Source: CAD feature listing. Evaluate the final solid. Frame: model axes, mm. A direction names the side the tool comes from. Give positions to 0.01 mm unless a question says otherwise; leave off trailing zeros. Order: outer loops, then holes, each group sorted by start corner. A loop starts at its lowest first (then second) coordinate and runs counter-clockwise, first axis right, second up. Notation, with made-up numbers: (-9, 21.5) - (14, 21.5) arc R12 cw to (14, 25.5) - close; hole circle Ø5 at (69.5, -11). An arc over 180 degrees is marked (long way). Answer as CSV lines item,"result".
```python
from build123d import *

# Parameters (mm, degrees)
SKETCH_W             = 47.4
SKETCH_H             = 2
PAD_DEPTH            = 10
SKETCH002_W          = 12
SKETCH002_H          = 10
PAD001_DEPTH         = 2.75
SKETCH003_R          = 1.65
POCKET_DEPTH         = 2.001
POCKET_DEPTH_BACK    = 2.751
POCKET001_DEPTH      = 2.001
POCKET001_DEPTH_BACK = 2.751


with BuildPart() as part:
    # Sketch → Pad (new body)
    with BuildSketch(Plane.XY):
        with Locations((0, 1)):
            Rectangle(SKETCH_W, SKETCH_H)
    extrude(amount=-PAD_DEPTH)

    # Sketch002 → Pad001 (join)
    with BuildSketch(Plane.XZ):
        with Locations((-6.6, -5)):
            Rectangle(SKETCH002_W, SKETCH002_H)
        with Locations((6.6, -5)):
            Rectangle(SKETCH002_W, SKETCH002_H)
    extrude(amount=PAD001_DEPTH)

    # Sketch003 → Pocket (cut, two sides)
    with BuildSketch(Plane.XZ) as pocket_sk:
        with Locations((-14.75, -5)):
            Circle(SKETCH003_R)
        with Locations((14.75, -5)):
            Circle(SKETCH003_R)
    extrude(amount=-POCKET_DEPTH, mode=Mode.SUBTRACT)
    extrude(pocket_sk.sketch, amount=POCKET_DEPTH_BACK, mode=Mode.SUBTRACT)

    # Sketch004 → Pocket001 (cut, two sides)
    with BuildSketch(Plane.XZ) as pocket001_sk:
        Polygon((-18.2, 0), (-23.7, -5.5), (-23.7, 0), align=None)
        Polygon((18.2, 0), (23.7, 0), (23.7, -5.5), align=None)
    extrude(amount=-POCKET001_DEPTH, mode=Mode.SUBTRACT)
    extrude(pocket001_sk.sketch, amount=POCKET001_DEPTH_BACK, mode=Mode.SUBTRACT)


solid = part.part
```
(1) Mould query, pull axis X, two halves, no side actions, for faces 4 (the flat face through (-12.6, -1, -5)), 5 (the flat face through (0, 0, -5)), 6 (the flat face through (21, 1, -2.8)), 7 (the flat face through (-7, -2.75, -5)). Classes: released by +X, released by -X, zero draft, split by the parting line, or undercut.
Completed:
face 4,"released by -X"
face 5,"undercut"
face 6,"released by +X"
face 7,"zero draft"
(2) Ray query, line 1 (Z direction, x = -14.75, y = 0.65); line 2 (X direction, y = -2.45, z = -3); line 3 (Y direction, x = 14, z = -6.75). Return the intervals inside material, ascending. Write a range as from..to.
Completed:
line 1,"-10..-6.65, -3.35..0"
line 2,"-12.6..-0.6, 0.6..12.6"
line 3,"0..2"
(3) Cut plane B-B (x = 14.75). Return loops of the section in (y, z), then the cut area to 3 significant figures.
Completed:
outline,"(0, -10) - (2, -10) - (2, -6.65) - (0, -6.65) - close; (0, -3.35) - (2, -3.35) - (2, 0) - (0, 0) - close"
area,"13.4 mm²"
(4) Cut plane D-D (y = 1.1). Return loops of the section in (x, z), then the cut area to 3 significant figures.
Completed:
outline,"(-23.7, -10) - (23.7, -10) - (23.7, -5.5) - (18.2, 0) - (-18.2, 0) - (-23.7, -5.5) - close; hole circle Ø3.3 at (-14.75, -5); hole circle Ø3.3 at (14.75, -5)"
area,"427 mm²"
(5) Access query for faces 1 (the flat face through (18, 0, -5)), 2 (the flat face through (0.6, -1, -5)), 3 (the flat face through (-18, 0, -5)). Directions: +Z, -Z, +X, -X, +Y, -Y. A direction counts if a zero-diameter tool reaches every point of the face in a straight line with its end or side. Return the directions, or none.
Completed:
face 1,"+Z, -Z, +X, -Y"
face 2,"+Z, -Z, -Y"
face 3,"+Z, -Z, -X, -Y"
(6) Contact query for flat-ended pins moving along their axis: pin 1 (3 mm diameter, centred on x = -18, z = -7, fed in from -Y); pin 2 (1.4 mm diameter, centred on y = -0.5, z = -3.5, fed in from -X); pin 3 (0.8 mm diameter, centred on y = -1, z = -6.5, fed in from +X); pin 4 (2 mm diameter, centred on x = 14.75, z = -5, fed in from -Y). Output: stop coordinate, or through.
Completed:
pin 1,"y = 0"
pin 2,"x = -22.19"
pin 3,"x = 12.6"
pin 4,"through"
(7) Cut plane A-A (z = -5). Return loops of the section in (x, y), then the cut area to 3 significant figures.
Completed:
outline,"(-23.2, 0) - (-16.4, 0) - (-16.4, 2) - (-23.2, 2) - close; (-13.1, 0) - (-12.6, 0) - (-12.6, -2.75) - (-0.6, -2.75) - (-0.6, 0) - (0.6, 0) - (0.6, -2.75) - (12.6, -2.75) - (12.6, 0) - (13.1, 0) - (13.1, 2) - (-13.1, 2) - close; (16.4, 0) - (23.2, 0) - (23.2, 2) - (16.4, 2) - close"
area,"146 mm²"
(8) Cut plane C-C (y = -1.65). Return loops of the section in (x, z), then the cut area to 3 significant figures.
Completed:
outline,"(-12.6, -10) - (-0.6, -10) - (-0.6, 0) - (-12.6, 0) - close; (0.6, -10) - (12.6, -10) - (12.6, 0) - (0.6, 0) - close"
area,"240 mm²"
